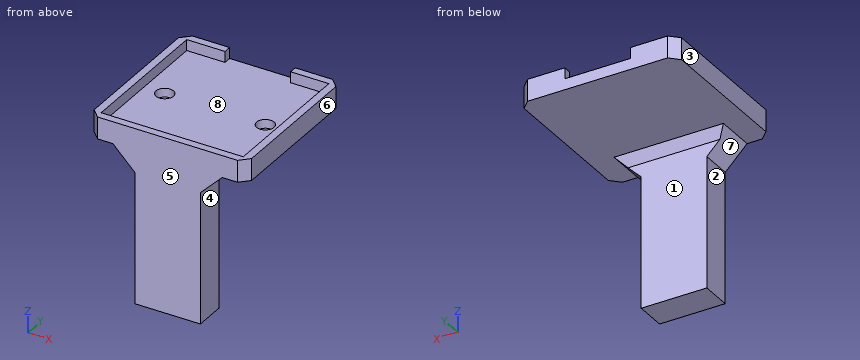
```python
from build123d import *

# Parameters (mm, degrees)
SKETCH3_W           = 36
SKETCH3_H           = 36
BOSS_EXTRUDE2_DEPTH = 5
SKETCH4_W           = 32.5
SKETCH4_H           = 32.5
SKETCH4_W_2         = 15
SKETCH4_H_2         = 1.75
CUT_EXTRUDE1_DEPTH  = 2.5
SKETCH6_W           = 35
SKETCH6_H           = 7
BOSS_EXTRUDE3_DEPTH = 7.5
CHAMFER1_SIZE       = 5
CHAMFER2_SIZE       = 2
SKETCH7_R           = 2
CUT_EXTRUDE2_DEPTH  = 2
CHAMFER3_SIZE       = 2


with BuildPart() as part:
    # Sketch3 → Boss-Extrude2 (new body)
    with BuildSketch(Plane.XY):
        Rectangle(SKETCH3_W, SKETCH3_H)
    extrude(amount=BOSS_EXTRUDE2_DEPTH)

    # Sketch4 → Cut-Extrude1 (cut)
    with BuildSketch(Plane.XY.offset(5)):
        Rectangle(SKETCH4_W, SKETCH4_H)
        with Locations((0, 17.125)):
            Rectangle(SKETCH4_W_2, SKETCH4_H_2)
    extrude(amount=-CUT_EXTRUDE1_DEPTH, mode=Mode.SUBTRACT)

    # Sketch6 → Boss-Extrude3 (add, symmetric)
    with BuildSketch(Plane(origin=(0, 0, 0), x_dir=(0, 0, -1), z_dir=(1, 0, 0))):
        with Locations((17.5, -14.5)):
            Rectangle(SKETCH6_W, SKETCH6_H)
    extrude(amount=BOSS_EXTRUDE3_DEPTH, both=True)

    # Chamfer1
    chamfer1_edges = [part.edges().sort_by_distance(p)[0] for p in [
        (-7.5, -14.5, 0),
        (7.5, -14.5, 0),
    ]]
    chamfer(chamfer1_edges, length=CHAMFER1_SIZE)

    # Chamfer2
    chamfer2_edges = [part.edges().sort_by_distance(p)[0] for p in [
        (18, -18, 2.5),
        (-18, -18, 2.5),
        (-18, 18, 2.5),
        (18, 18, 2.5),
    ]]
    chamfer(chamfer2_edges, length=CHAMFER2_SIZE)

    # Sketch7 → Cut-Extrude2 (cut)
    with BuildSketch(Plane.XY.offset(2.5)):
        with Locations((-11.5, 0)):
            Circle(SKETCH7_R)
        with Locations(Location((11.5, 0, 0), (0, 0, 180))):
            Circle(SKETCH7_R)
    extrude(amount=-CUT_EXTRUDE2_DEPTH, mode=Mode.SUBTRACT)

    # Chamfer3
    chamfer3_edges = [part.edges().sort_by_distance(p)[0] for p in [
        (0, -11, 0),
    ]]
    chamfer(chamfer3_edges, length=CHAMFER3_SIZE)


solid = part.part
```
Can you work these out from the model? Positions are in its coordinate system, mm. Face numbers are marked on the shaded views. A direction names the side the tool comes from. Round coordinates to 2 decimals unless told otherwise and drop trailing zeros. Loops run counter-clockwise (first coordinate to the right, second up) from the corner with the lowest first, then second, coordinate; pieces in that order, holes last. Notation, with made-up numbers: M 3.5,30 L 27.5,30 A35 ccw 27.5,66 Z; hole C 32,83.25 d8. An arc over 180 degrees is marked long. Answer as a JSON object with one key per item and string values. Group by question number.
Q1. Will these pins go through, and if not, where does the flat tip stop? pin 1 (10 mm diameter, centred on x = -9, y = 0, fed in from +Z); pin 2 (3 mm diameter, centred on x = -5.5, z = 3.5, fed in from +Y); pin 3 (4 mm diameter, centred on x = 6, z = -24.5, fed in from +Y); pin 4 (0.9 mm diameter, centred on y = 17, z = 4, fed in from -X).
Q2. We'd pull the mould along X, two halves only. Please class the marked faces 5, 6, 7 and 8: +X half, -X half, draft (parallel to the pull), parting line (faces both ways), or undercut.
Q3. Imagine slicing it at D-D, the plane y = 6. Please give me the cut outline in (x, z).
Q4. Imagine slicing it at A-A, the plane x = -11.5. Please give me the cut outline in (y, z), then the cut area to 4 significant figures.
Q5. On a 3-axis mill with a long thin cutter (end or side, diameter ignored), from which of +Z, -Z, +X, -X, +Y, -Y can I reach the whole of each face in a straight line? I mean the marked faces 1, 2, 3 and 4. Say none if no direction works.
Q6. Please list where these lines run through material, in increasing order: L1, parallel to Y at x = -11.5, z = 1.3; L2, parallel to Y at x = 0, z = -4.5; L3, parallel to Z at x = -4.5, y = 12.5.
Q7. Imagine slicing it at C-C, the plane z = -10. Please give me the cut outline in (x, y).
Q8. Imagine slicing it at B-B, the plane y = -14. Please give me the cut outline in (x, z), then the cut area to 3 significant figures.
Findings:
{
 "1": {"pin 1": "stops at z = 2.5", "pin 2": "stops at y = 18", "pin 3": "stops at y = -11", "pin 4": "stops at x = -17.45"},
 "2": {"face 5": "draft", "face 6": "+X half", "face 7": "-X half", "face 8": "undercut"},
 "3": {"outline": "M -18,0 L 18,0 L 18,5 L 16.25,5 L 16.25,2.5 L -16.25,2.5 L -16.25,5 L -18,5 Z"},
 "4": {"outline": "M -18,-1 L -10,-1 L -9,0 L 18,0 L 18,5 L 16.25,5 L 16.25,2.5 L 2,2.5 L 2,0.5 L -2,0.5 L -2,2.5 L -16.25,2.5 L -16.25,5 L -18,5 Z", "area": "99.25 mm2"},
 "5": {"face 1": "-Z, +X, -X, +Y", "face 2": "-Z, -X, +Y, -Y", "face 3": "+Z, -Z, -X, +Y, -Y", "face 4": "-Z, +X, +Y, -Y"},
 "6": {"L1": "y = -18 to -2, 2 to 18", "L2": "y = -18 to -11", "L3": "z = 0 to 2.5"},
 "7": {"outline": "M -7.5,-18 L 7.5,-18 L 7.5,-11 L -7.5,-11 Z"},
 "8": {"outline": "M -18,0 L -12.5,0 L -7.5,-5 L -7.5,-35 L 7.5,-35 L 7.5,-5 L 12.5,0 L 18,0 L 18,5 L 16.25,5 L 16.25,2.5 L -16.25,2.5 L -16.25,5 L -18,5 Z", "area": "649 mm2"}
}
